```python
from build123d import *

# Parameters (mm, degrees)
F0_W     = 42
F0_H     = 12
F1_DEPTH = 10
F2_W     = 8
F2_H     = 12
F3_DEPTH = 105
F4_W     = 42
F4_H     = 12
F5_DEPTH = 10
F6_W     = 58
F6_H     = 10
F7_DEPTH = 3
F8_R     = 1.5
F9_DEPTH = 9.9999997765


# Not quite as in the source:
# - a pattern or mirror of a feature is missing from the dataset's text; its kind, count and spacing are read off the source's solid


with BuildPart() as f1:
    # F0 (on Top) → F1 (new body)
    with BuildSketch(Plane.XY):
        Rectangle(F0_W, F0_H)
    extrude(amount=F1_DEPTH)

    # F2 (on face) → F3 (join)
    with BuildSketch(Plane.XY.offset(10)):
        with Locations((-17, 0)):
            Rectangle(F2_W, F2_H)
        with Locations((17, 0)):
            Rectangle(F2_W, F2_H)
    extrude(amount=F3_DEPTH)

    # F4 (on face) → F5 (join)
    with BuildSketch(Plane.XY.offset(115)):
        Rectangle(F4_W, F4_H)
    extrude(amount=F5_DEPTH)

    # F6 (on face) → F7 (join)
    with BuildSketch(Plane.XZ.offset(6)):
        with Locations((0, 5)):
            Rectangle(F6_W, F6_H)
    f7 = extrude(amount=F7_DEPTH)

    # F7_copies: F7 across plane
    add(f7.mirror(Plane.ZX))

    # F8 (on face) → F9 (cut)
    with BuildSketch(Plane.XY.offset(10)):
        with Locations((-7, 0)):
            Circle(F8_R)
        with Locations((1, 0)):
            Circle(F8_R)
        with Locations((9, 0)):
            Circle(F8_R)
    extrude(amount=-F9_DEPTH, mode=Mode.SUBTRACT)


solid = f1.part
```
Geometry: final body of the model. Coordinates: model frame, mm. A direction names the side the tool comes from. Give positions to 0.01 mm unless a question says otherwise; leave off trailing zeros. Order: outer loops, then holes, each group sorted by start corner. A loop starts at its lowest first (then second) coordinate and runs counter-clockwise, first axis right, second up. Notation, with made-up numbers: M -2.5,-9.75 L 43.5,-9.75 A17 cw 43.5,15.25 Z; hole C 15.25,-6.75 d6. An arc over 180 degrees is marked long. Answer as CSV lines item,"result". Start each with the question number.
1) Line query: line 1 (Z direction, x = 12, y = -3.25); line 2 (Y direction, x = 1, z = 6); line 3 (X direction, y = -1.75, z = 68). Output: solid intervals per line, ascending. Write a range as from..to.
2) Cut plane D-D (x = -24). Output: boundary loops of the cut face in (y, z), then the cut area to 3 significant figures.
3) Cut plane A-A (z = 95.5). Output: boundary loops of the cut face in (x, y).
4) Cut plane C-C (y = 0). Output: boundary loops of the cut face in (x, z).
5) Cut plane B-B (x = 1). Output: boundary loops of the cut face in (y, z).
6) First-contact query: P1, Ø3.5, axis at y = 2.5, z = 77.5, coming from the -X side; P2, Ø10, axis at y = 0, z = 97.5, coming from the +X side; P3, Ø1.8, axis at x = 1, y = 0, coming from the -Z side. Flat tips, straight axial feed; report the tip coordinate or a pass-through.
7) Mould query, pull axis X, two halves, no side actions, for faces 5 (the flat face through (0, -2, 10)), 6 (the flat face through (-21, 0, 62)), 7 (the flat face through (29, -7, 5)), 8 (the flat face through (25, 6, 5)). Classes: +X half, -X half, draft (parallel to the pull), parting line (faces both ways), or undercut.
8) Set-up query: faces 1 (the flat face through (-25, 6, 5)), 2 (the cylindrical face through (2.386, -0.575, 5.07)), 3 (the flat face through (25, -6, 5)), 4 (the flat face through (-13, 0, 62)). Return all of +Z, -Z, +X, -X, +Y, -Y with unobstructed straight access to the full face (end or side cutting, diameter ignored); none if empty.
Findings below:
1,line 1,"z = 0..10, 115..125"
1,line 2,"y = -9..-1.5, 1.5..9"
1,line 3,"x = -21..-13, 13..21"
2,outline,"M -9,0 L -6,0 L -6,10 L -9,10 Z; M 6,0 L 9,0 L 9,10 L 6,10 Z"
2,area,"60.0 mm²"
3,outline,"M -21,-6 L -13,-6 L -13,6 L -21,6 Z; M 13,-6 L 21,-6 L 21,6 L 13,6 Z"
4,outline,"M -21,0 L -8.5,0 L -8.5,10 L -13,10 L -13,115 L 13,115 L 13,10 L 10.5,10 L 10.5,0 L 21,0 L 21,125 L -21,125 Z; M -5.5,0 L -0.5,0 L -0.5,10 L -5.5,10 Z; M 2.5,0 L 7.5,0 L 7.5,10 L 2.5,10 Z"
5,outline,"M -9,0 L -1.5,0 L -1.5,10 L -9,10 Z; M -6,115 L 6,115 L 6,125 L -6,125 Z; M 1.5,0 L 9,0 L 9,10 L 1.5,10 Z"
6,P1,"stops at x = -21"
6,P2,"stops at x = 21"
6,P3,"stops at z = 115"
7,face 5,"undercut"
7,face 6,"-X half"
7,face 7,"+X half"
7,face 8,"draft"
8,face 1,"+Z, -Z, -X"
8,face 2,"-Z"
8,face 3,"+Z, -Z, +X"
8,face 4,"+Y, -Y"
